Part model, mm, in its own coordinate system. Face numbers are marked on the shaded views. A direction names the side the tool comes from. Coordinates: 2 decimals unless noted, no trailing zeros. Loops run counter-clockwise (first coordinate to the right, second up) from the corner with the lowest first, then second, coordinate; pieces in that order, holes last. Notation, with made-up numbers: (-12.5, -16) - (11.5, -16) arc R21 ccw to (11.5, 2) - close; hole circle Ø10 at (86, 11). An arc over 180 degrees is marked (long way). Use a Markdown table: item, result. Add a question column.
1) Band-saw the part on B-B (z = -6.5). Give the cut face in (x, y) (3 decimals).
2) Band-saw the part on D-D (z = 10). Give the cut face in (x, y) (3 decimals).
3) Probe probe 1 along Z at (x, y) = (-48.5, -27.5); probe 2 along Y at (x, z) = (-5.5, -24) (3 decimals); probe 3 along Y at (x, z) = (-63.5, -35) (3 decimals). List the from-to ranges inside material, lowest first. Write a range as [from, to].
4) Band-saw the part on C-C (y = -23.5). Give the cut face in (x, z) (1 decimal), plus the area to 3 significant figures.
5) Drop flat-ended pins along their axis: P1, Ø12.5, axis at x = 5, y = -26.5, coming from the +Z side; P2, Ø1.5, axis at y = -21, z = 17, coming from the +X side; P3, Ø20.5, axis at x = 8.24, z = -10.16, coming from the -Y side. Give the stop position or say it passes through.
6) Pull direction X, two halves, no side cores. Call the marked faces 1, 2 and 3: +X half, -X half, draft (parallel to the pull), parting line (faces both ways), or undercut.
7) Band-saw the part on A-A (x = -61). Give the cut face in (y, z) (3 decimals).
8) Tool access for the marked faces 4, 5 and 6: list every direction of +Z, -Z, +X, -X, +Y, -Y with a clear straight run to the whole face (end or side of a thin tool).
from build123d import *

# Parameters (mm, degrees)
F0_W      = 107.95
F0_H      = 76.2
F1_DEPTH  = 41.275
F2_W      = 107.95
F2_H      = 60.325
F3_DEPTH  = 9.525
F4_W      = 53.975
F4_H      = 25.4
F5_DEPTH  = 31.751
F6_W      = 15.875
F6_H      = 50.8
F7_DEPTH  = 107.951
F8_W      = 15.875
F8_H      = 9.525
F9_DEPTH  = 53.976
F10_R     = 7.9375
F11_DEPTH = 31.751


with BuildPart() as f1:
    # F0 (on Front) → F1 (new body)
    with BuildSketch(Plane.XZ):
        with Locations((-20.33008, -8.164287)):
            Rectangle(F0_W, F0_H)
    extrude(amount=F1_DEPTH)

    # F2 (on face) → F3 (cut)
    with BuildSketch(Plane.XZ.offset(41.275)):
        with Locations((-20.33008, -0.226787)):
            Rectangle(F2_W, F2_H)
    extrude(amount=-F3_DEPTH, mode=Mode.SUBTRACT)

    # F4 (on face) → F5 (cut, through all)
    with BuildSketch(Plane.XZ.offset(31.75)):
        with Locations((6.65742, 17.235713)):
            Rectangle(F4_W, F4_H)
    extrude(amount=-F5_DEPTH, mode=Mode.SUBTRACT)

    # F6 (on face) → F7 (cut, through all)
    with BuildSketch(Plane.YZ.offset(33.64492)):
        with Locations((-7.9375, -20.864287)):
            Rectangle(F6_W, F6_H)
    extrude(amount=-F7_DEPTH, mode=Mode.SUBTRACT)

    # F8 (on face) → F9 (cut, through all)
    with BuildSketch(Plane.YZ.offset(-20.33008)):
        with Locations((-7.9375, 9.298213)):
            Rectangle(F8_W, F8_H)
    extrude(amount=-F9_DEPTH, mode=Mode.SUBTRACT)

    # F10 (on face) → F11 (cut, through all)
    with BuildSketch(Plane.XZ.offset(31.75)):
        with Locations((-48.90508, -9.899196)):
            Circle(F10_R)
        with Locations((8.24492, -10.156629)):
            Circle(F10_R)
    extrude(amount=-F11_DEPTH, mode=Mode.SUBTRACT)


solid = f1.part
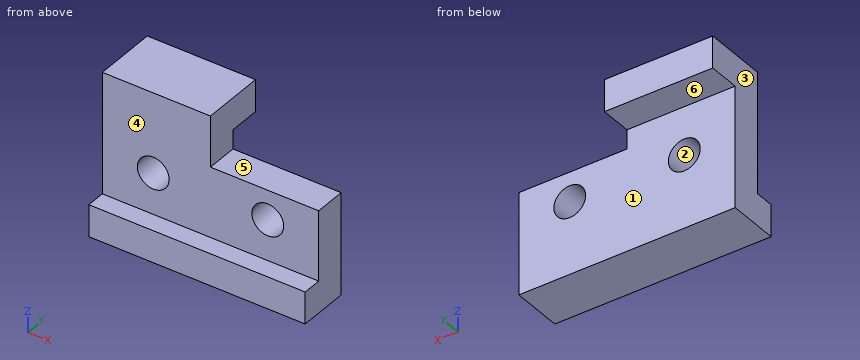
Answer block:
| question | item | result |
|---|---|---|
| 1 | outline | (-74.305, -31.75) - (-56.078, -31.75) - (-56.078, -15.875) - (-74.305, -15.875) - close; (-41.732, -31.75) - (1.2, -31.75) - (1.2, -15.875) - (-41.732, -15.875) - close; (15.29, -31.75) - (33.645, -31.75) - (33.645, -15.875) - (15.29, -15.875) - close |
| 2 | outline | (-74.305, -31.75) - (-20.33, -31.75) - (-20.33, -15.875) - (-74.305, -15.875) - close |
| 3 | probe 1 | [-46.26, -17.83], [-1.97, 29.94] |
| 3 | probe 2 | [-31.75, -15.875] |
| 3 | probe 3 | [-41.275, -15.875] |
| 4 | outline | (-74.3, -46.3) - (33.6, -46.3) - (33.6, 4.5) - (-20.3, 4.5) - (-20.3, 29.9) - (-74.3, 29.9) - close; hole circle Ø15.9 at (-48.9, -9.9); hole circle Ø15.9 at (8.2, -10.2) |
| 4 | area | 6,460 mm2 |
| 5 | P1 | z = 4.54 |
| 5 | P2 | x = -20.33 |
| 5 | P3 | y = -31.75 |
| 6 | face 1 | draft |
| 6 | face 2 | undercut |
| 6 | face 3 | -X half |
| 7 | outline | (-41.275, -46.264) - (-15.875, -46.264) - (-15.875, 14.061) - (0, 14.061) - (0, 29.936) - (-31.75, 29.936) - (-31.75, -30.389) - (-41.275, -30.389) - close |
| 8 | face 4 | +Z, +X, -X, -Y |
| 8 | face 5 | +Z, +X, +Y, -Y |
| 8 | face 6 | -Z, +X, -X, +Y |
